```python
from build123d import *

# Parameters (mm, degrees)
SKETCH_1_R               = 31.5
SKETCH_1_R_2             = 18.25
EXTRUDE_1_DEPTH          = 3
CHAMFER_2_SIZE           = 1
CHAMFER_3_SIZE           = 0.5
SKETCH_2_R               = 1.6
CUT_EXTRUDE_1_DEPTH      = 4
PATTERN_CIRCULAR_1_COUNT = 4


with BuildPart() as part:
    # Sketch 1 → Extrude 1 (new body)
    with BuildSketch(Plane.XY):
        Circle(SKETCH_1_R)
        Circle(SKETCH_1_R_2, mode=Mode.SUBTRACT)
    extrude(amount=EXTRUDE_1_DEPTH)

    # Chamfer 2
    chamfer_2_edges = [part.edges().sort_by_distance(p)[0] for p in [
        (-18.25, 0, 3),
    ]]
    chamfer(chamfer_2_edges, length=CHAMFER_2_SIZE)

    # Chamfer 3
    chamfer_3_edges = [part.edges().sort_by_distance(p)[0] for p in [
        (-31.5, 0, 3),
    ]]
    chamfer(chamfer_3_edges, length=CHAMFER_3_SIZE)

    # Sketch 2 → Cut-Extrude 1 (cut, through all)
    with BuildSketch(Plane(origin=(0, 0, 0), x_dir=(-1, 0, 0), z_dir=(0, 0, -1))):
        with Locations((-16.263455967, 16.263455967)):
            Circle(SKETCH_2_R)
    cut_extrude_1 = extrude(amount=-CUT_EXTRUDE_1_DEPTH, mode=Mode.SUBTRACT)

    # Pattern Circular 1: Cut-Extrude 1 ×4 about axis
    pattern_circular_1_axis = Axis((0, 0, 0), (0, 0, 1))
    for i in range(1, PATTERN_CIRCULAR_1_COUNT):
        add(cut_extrude_1.rotate(pattern_circular_1_axis, i * 360 / PATTERN_CIRCULAR_1_COUNT), mode=Mode.SUBTRACT)


solid = part.part
```
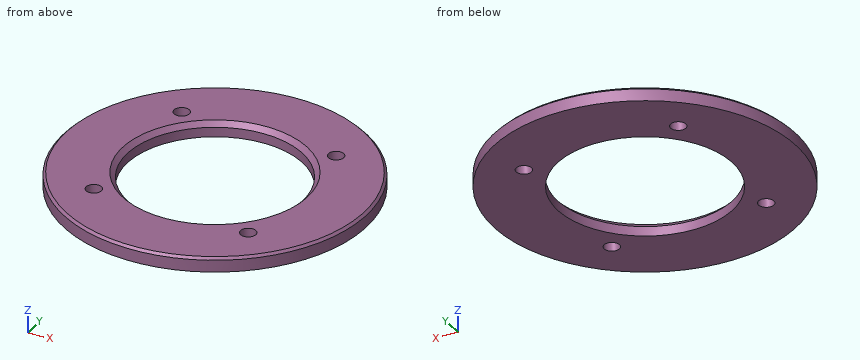
Geometry check sheet. Reference: the model listing, model coordinates, mm. Coordinates: 2 decimals unless noted, no trailing zeros. Write each loop counter-clockwise with the first axis right and the second up, starting at its lowest first coordinate (ties: lowest second). Pieces come first, ordered by that corner, then holes. Notation, with made-up numbers: M -21.75,82 L 1.25,82 A22 cw 1.25,110 Z; hole C 6.5,28 d1. An arc over 180 degrees is marked long. Answer as a JSON object with one key per item and string values.
1. Section check C-C, the plane z = 1.4. Enter the section's corners in (x, y), plus the area to 3 significant figures.
Answers below:
{"outline": "C 0,0 d63; hole C 0,0 d36.5; hole C -16.26,-16.26 d3.2; hole C -16.26,16.26 d3.2; hole C 16.26,-16.26 d3.2; hole C 16.26,16.26 d3.2", "area": "2,040 mm²"}
2. Section check A-A, the plane y = 0. Enter the section's corners in (x, z), plus the area to 4 significant figures.
Answers below:
{"outline": "M -31.5,0 L -18.25,0 L -18.25,2 L -19.25,3 L -31,3 L -31.5,2.5 Z; M 18.25,0 L 31.5,0 L 31.5,2.5 L 31,3 L 19.25,3 L 18.25,2 Z", "area": "78.25 mm²"}
3. Go/stop test with flat-tipped pins: pin 1 Ø1.5 at (x, z) = (8.5, 1) entering from +Y; pin 2 Ø1.5 at (y, z) = (-10, 1) entering from -X. Record where each tip stops, or that it passes through.
Answers below:
{"pin 1": "stops at y = 30.53", "pin 2": "stops at x = -30.11"}
4. Scan lines: L1, parallel to X at y = -12, z = 1.85; L2, parallel to Y at x = -3.5, z = 1.05; L3, parallel to Y at x = -9, z = 0.45. Record each from-to range of solid material in increasing order.
Answers below:
{"L1": "x = -29.12 to -13.75, 13.75 to 29.12", "L2": "y = -31.3 to -17.91, 17.91 to 31.3", "L3": "y = -30.19 to -15.88, 15.88 to 30.19"}
